Model file for the job. Use its own axes, mm. Face numbers are marked on the shaded views. Coordinates: 2 decimals unless noted, no trailing zeros. Write each loop counter-clockwise with the first axis right and the second up, starting at its lowest first coordinate (ties: lowest second). Pieces come first, ordered by that corner, then holes. Notation, with made-up numbers: (50, -16.5) -> (69, -16.5) arc R5 ccw to (69, -10.5) -> close; hole circle Ø5 at (-18.75, 88.5). An arc over 180 degrees is marked (long way). Answer as a JSON object with one key per item and string values. Group by question number.
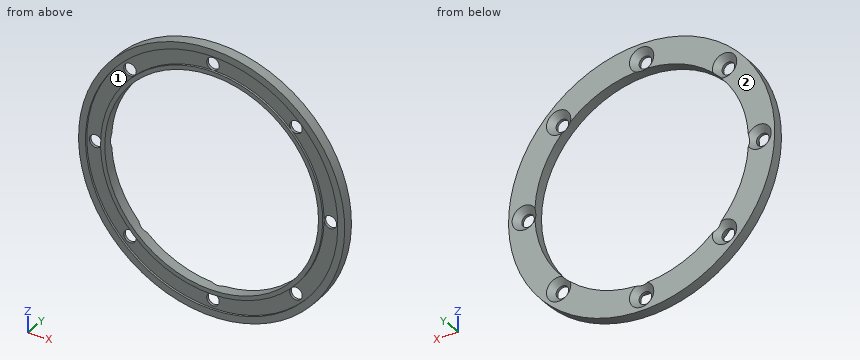
from build123d import *

# Parameters (mm, degrees)
SKETCH_1_R               = 31.75
SKETCH_1_R_2             = 25.5
EXTRUDE_1_DEPTH          = 2.5
SKETCH_2_R               = 1.5
CUT_EXTRUDE_1_DEPTH      = 10
SKETCH_3_R               = 30.1
SKETCH_3_R_2             = 26.5
CUT_EXTRUDE_2_DEPTH      = 0.5
HOLE_WIZARD_1_AT_2_COUNT = 2
HOLE_WIZARD_1_AT_2_PITCH = 21.430272212
HOLE_WIZARD_1_AT_3_COUNT = 2
HOLE_WIZARD_1_AT_3_PITCH = 39.597979746
HOLE_WIZARD_1_AT_4_COUNT = 2
HOLE_WIZARD_1_AT_4_PITCH = 51.737253821
HOLE_WIZARD_1_AT_5_COUNT = 2
HOLE_WIZARD_1_AT_5_PITCH = 56
HOLE_WIZARD_1_AT_6_COUNT = 2
HOLE_WIZARD_1_AT_6_PITCH = 39.597979746
HOLE_WIZARD_1_AT_7_COUNT = 2
HOLE_WIZARD_1_AT_7_PITCH = 21.430272212
HOLE_WIZARD_1_AT_8_COUNT = 2
HOLE_WIZARD_1_AT_8_PITCH = 51.737253821


with BuildPart() as part:
    # 草图1 → 凸台-拉伸1 (new body)
    with BuildSketch(Plane(origin=(0, 0, 0), x_dir=(1, 0, 0), z_dir=(0, 1, 0))):
        with Locations(Location((0, 0, 0), (0, 0, 270))):
            Circle(SKETCH_1_R)
        with Locations(Location((0, 0, 0), (0, 0, 270))):
            Circle(SKETCH_1_R_2, mode=Mode.SUBTRACT)
    extrude(amount=EXTRUDE_1_DEPTH)

    # 草图2 → 切除-拉伸1 (cut)
    with BuildSketch(Plane.XZ):
        with Locations(Location((0, -28, 0), (0, 0, 270))):
            Circle(SKETCH_2_R)
        with Locations(Location((-19.798989873, -19.798989873, 0), (0, 0, 270))):
            Circle(SKETCH_2_R)
        with Locations(Location((-28, 0, 0), (0, 0, 270))):
            Circle(SKETCH_2_R)
        with Locations(Location((-19.798989873, 19.798989873, 0), (0, 0, 270))):
            Circle(SKETCH_2_R)
        with Locations(Location((0, 28, 0), (0, 0, 270))):
            Circle(SKETCH_2_R)
        with Locations(Location((19.798989873, 19.798989873, 0), (0, 0, 270))):
            Circle(SKETCH_2_R)
        with Locations(Location((28, 0, 0), (0, 0, 270))):
            Circle(SKETCH_2_R)
        with Locations(Location((19.798989873, -19.798989873, 0), (0, 0, 270))):
            Circle(SKETCH_2_R)
    extrude(amount=-CUT_EXTRUDE_1_DEPTH, mode=Mode.SUBTRACT)

    # 草图3 → 切除-拉伸2 (cut)
    with BuildSketch(Plane.XZ):
        with Locations(Location((0, 0, 0), (0, 0, 270))):
            Circle(SKETCH_3_R)
        with Locations(Location((0, 0, 0), (0, 0, 270))):
            Circle(SKETCH_3_R_2, mode=Mode.SUBTRACT)
    extrude(amount=-CUT_EXTRUDE_2_DEPTH, mode=Mode.SUBTRACT)

    # 草图4 → 打孔尺寸(%根据十字)槽沉头木螺钉的类型1 (revolve, cut)
    with BuildSketch(Plane(origin=(0, 2.5, -28), x_dir=(0, 0, 1), z_dir=(1, 0, 0))):
        Polygon((0, 0), (0, 2.5), (1.5, 2.5), (1.5, 1.4), (2.9, 0), align=None)
    hole_wizard_1 = revolve(axis=Axis((0, 8.85, -28), (0, -1, 0)), mode=Mode.SUBTRACT)

    # 打孔尺寸(%根据十字)槽沉头木螺钉的类型1 at 2: 打孔尺寸(%根据十字)槽沉头木螺钉的类型1 ×2
    with Locations(*[Vector(0.9238795325112867, 0, 0.3826834323650898) * (i * HOLE_WIZARD_1_AT_2_PITCH) for i in range(1, HOLE_WIZARD_1_AT_2_COUNT)]):
        add(hole_wizard_1, mode=Mode.SUBTRACT)

    # 打孔尺寸(%根据十字)槽沉头木螺钉的类型1 at 3: 打孔尺寸(%根据十字)槽沉头木螺钉的类型1 ×2
    with Locations(*[Vector(0.7071067811865476, 0, 0.7071067811865476) * (i * HOLE_WIZARD_1_AT_3_PITCH) for i in range(1, HOLE_WIZARD_1_AT_3_COUNT)]):
        add(hole_wizard_1, mode=Mode.SUBTRACT)

    # 打孔尺寸(%根据十字)槽沉头木螺钉的类型1 at 4: 打孔尺寸(%根据十字)槽沉头木螺钉的类型1 ×2
    with Locations(*[Vector(0.3826834323650897, 0, 0.9238795325112867) * (i * HOLE_WIZARD_1_AT_4_PITCH) for i in range(1, HOLE_WIZARD_1_AT_4_COUNT)]):
        add(hole_wizard_1, mode=Mode.SUBTRACT)

    # 打孔尺寸(%根据十字)槽沉头木螺钉的类型1 at 5: 打孔尺寸(%根据十字)槽沉头木螺钉的类型1 ×2
    with Locations(*[(0, 0, i * HOLE_WIZARD_1_AT_5_PITCH) for i in range(1, HOLE_WIZARD_1_AT_5_COUNT)]):
        add(hole_wizard_1, mode=Mode.SUBTRACT)

    # 打孔尺寸(%根据十字)槽沉头木螺钉的类型1 at 6: 打孔尺寸(%根据十字)槽沉头木螺钉的类型1 ×2
    with Locations(*[Vector(-0.7071067811865476, 0, 0.7071067811865476) * (i * HOLE_WIZARD_1_AT_6_PITCH) for i in range(1, HOLE_WIZARD_1_AT_6_COUNT)]):
        add(hole_wizard_1, mode=Mode.SUBTRACT)

    # 打孔尺寸(%根据十字)槽沉头木螺钉的类型1 at 7: 打孔尺寸(%根据十字)槽沉头木螺钉的类型1 ×2
    with Locations(*[Vector(-0.9238795325112868, 0, 0.3826834323650896) * (i * HOLE_WIZARD_1_AT_7_PITCH) for i in range(1, HOLE_WIZARD_1_AT_7_COUNT)]):
        add(hole_wizard_1, mode=Mode.SUBTRACT)

    # 打孔尺寸(%根据十字)槽沉头木螺钉的类型1 at 8: 打孔尺寸(%根据十字)槽沉头木螺钉的类型1 ×2
    with Locations(*[Vector(-0.3826834323650898, 0, 0.9238795325112867) * (i * HOLE_WIZARD_1_AT_8_PITCH) for i in range(1, HOLE_WIZARD_1_AT_8_COUNT)]):
        add(hole_wizard_1, mode=Mode.SUBTRACT)


solid = part.part
(1) Wall check: probe 1 along X at (y, z) = (0.4, 0); probe 2 along X at (y, z) = (0.35, -6.5); probe 3 along Y at (x, z) = (-24, -14). Give the ranges that are in metal, low to high.
(2) Pin check, flat tips, straight feed: pin 1 (4 mm diameter, centred on x = 19.8, z = -19.8, fed in from +Y); pin 2 (4 mm diameter, centred on x = 0, z = 28, fed in from -Y); pin 3 (1.5 mm diameter, centred on y = 1, z = -16.5, fed in from -X). Stop position of each tip, or through.
(3) Cut at A-A on x = -13. List the corners of the cut face in (y, z), plus the area to 3 significant figures.
(4) Cut at D-D on z = 28. List the corners of the cut face in (x, y), plus the area to 3 significant figures.
(5) Pull direction X, two halves, no side cores. Call the marked faces 1 and 2: released by +X, released by -X, zero draft, split by the parting line, or undercut.
(6) Cut at C-C on x = 28. List the corners of the cut face in (y, z), plus the area to 3 significant figures.
(7) Cut at B-B on z = 12. List the corners of the cut face in (x, y), plus the area to 3 significant figures.
Results found:
{
 "1": {"probe 1": "x = -31.75 to -30.1, -26.5 to -25.5, 25.5 to 26.5, 30.1 to 31.75", "probe 2": "x = -31.08 to -29.39, -25.69 to -24.66, 24.66 to 25.69, 29.39 to 31.08", "probe 3": "y = 0.5 to 2.5"},
 "2": {"pin 1": "stops at y = 1.6", "pin 2": "stops at y = 0", "pin 3": "stops at x = -27.57"},
 "3": {"outline": "(0, -28.97) -> (2.5, -28.97) -> (2.5, -21.94) -> (0, -21.94) -> (0, -23.09) -> (0.5, -23.09) -> (0.5, -27.15) -> (0, -27.15) -> close; (0, 21.94) -> (2.5, 21.94) -> (2.5, 28.97) -> (0, 28.97) -> (0, 27.15) -> (0.5, 27.15) -> (0.5, 23.09) -> (0, 23.09) -> close", "area": "31.1 mm²"},
 "4": {"outline": "(-14.97, 0) -> (-11.05, 0) -> (-11.05, 0.5) -> (-1.5, 0.5) -> (-1.5, 1.1) -> (-2.9, 2.5) -> (-14.97, 2.5) -> close; (1.5, 0.5) -> (11.05, 0.5) -> (11.05, 0) -> (14.97, 0) -> (14.97, 2.5) -> (2.9, 2.5) -> (1.5, 1.1) -> close", "area": "55.8 mm²"},
 "5": {"face 1": "undercut", "face 2": "zero draft"},
 "6": {"outline": "(0, -14.97) -> (2.5, -14.97) -> (2.5, -2.9) -> (1.1, -1.5) -> (0.5, -1.5) -> (0.5, -11.05) -> (0, -11.05) -> close; (0, 11.05) -> (0.5, 11.05) -> (0.5, 1.5) -> (1.1, 1.5) -> (2.5, 2.9) -> (2.5, 14.97) -> (0, 14.97) -> close", "area": "55.8 mm²"},
 "7": {"outline": "(-29.39, 0) -> (-27.6, 0) -> (-27.6, 0.5) -> (-23.63, 0.5) -> (-23.63, 0) -> (-22.5, 0) -> (-22.5, 2.5) -> (-29.39, 2.5) -> close; (22.5, 0) -> (23.63, 0) -> (23.63, 0.5) -> (27.6, 0.5) -> (27.6, 0) -> (29.39, 0) -> (29.39, 2.5) -> (22.5, 2.5) -> close", "area": "30.5 mm²"}
}
